Input: part model. Units: mm. Frame: model coordinates. Face numbers are marked on the shaded views. A direction names the side the tool comes from. Coordinates: 2 decimals unless noted, no trailing zeros. Write each loop counter-clockwise with the first axis right and the second up, starting at its lowest first coordinate (ties: lowest second). Pieces come first, ordered by that corner, then holes.
Autodesk Inventor part; units mm, degrees
ref_plane "YZ Plane" through (0, 0, 0) normal (1, 0, 0) x (0, 1, 0)
ref_plane "XZ Plane" through (0, 0, 0) normal (0, 1, 0) x (-1, 0, 0)
ref_plane "XY Plane" through (0, 0, 0) normal (0, 0, 1) x (1, 0, 0)
ref_plane "Work Plane1" through (0, 0, 0) normal (0, 0, 1) x (1, 0, 0)
sketch "Sketch1" plane through (0, 0, 0) normal (0, 0, 1) x (1, 0, 0)
  circle A0 centre (0, 25) radius 1.95 construction
  circle A1 centre (-25, 0) radius 1.95 construction
  circle A2 centre (-25, -25) radius 1.95 construction
  circle A3 centre (25, 25) radius 1.95 construction
  circle A4 centre (25, -25) radius 1.95 construction
  circle A5 centre (-25, 25) radius 1.95 construction
  circle A6 centre (25, 0) radius 1.95 construction
  circle A7 centre (0, -25) radius 1.95 construction
  line L0 (-28, 30) -> (-30, 28) construction
  line L1 (-30, 28) -> (-30, -28) construction
  line L2 (-30, -28) -> (-28, -30) construction
  line L3 (-28, -30) -> (28, -30) construction
  line L4 (28, -30) -> (30, -28) construction
  line L5 (30, -28) -> (30, 28) construction
  line L6 (30, 28) -> (28, 30) construction
  line L7 (28, 30) -> (-28, 30) construction
  circle A8 centre (35, -56) radius 1 construction
  circle A9 centre (5, -48.5) radius 1 construction
  circle A10 centre (5, -64.5) radius 1.0474 construction
  circle A11 centre (-5, -64.5) radius 1 construction
  circle A12 centre (-5, -56) radius 1 construction
  circle A13 centre (-5, -48.5) radius 1 construction
  circle A14 centre (5, -56) radius 1 construction
  circle A15 centre (35, -48) radius 1 construction
  circle A16 centre (35, -64) radius 1 construction
  line L8 (38, -40) -> (38, -72) construction
  line L9 (38, -40) -> (-10, -40) construction
  line L10 (-10, -72) -> (-10, -40) construction
  line L11 (38, -72) -> (-10, -72) construction
  line L12 (38, -71) -> (38, -41) construction
  line L13 (38, -71) -> (48, -71) construction
  line L14 (48, -41) -> (48, -71) construction
  line L15 (38, -41) -> (48, -41) construction
  line L16 (56, -75) -> (-52.5, -75)
  line L17 (-52.5, -75) -> (-52.5, -30)
  line L18 (-52.5, -30) -> (56, -30)
  line L19 (56, -30) -> (56, -75)
  line L20 (-40, -41.1445) -> (-40, -68) construction
  line L21 (-41, -39.0927) -> (-41, -47.7587) construction
  line L22 (-41, -39.0927) -> (-46.5, -39.0927) construction
  line L23 (-46.5, -47.7587) -> (-46.5, -39.0927) construction
  line L24 (-41, -47.7587) -> (-46.5, -47.7587) construction
  line L25 (-41, -60.5) -> (-41, -64) construction
  line L26 (-41, -60.5) -> (-46.5, -60.5) construction
  line L27 (-46.5, -64) -> (-46.5, -60.5) construction
  line L28 (-41, -64) -> (-46.5, -64) construction
  line L29 (64, 30) -> (-96, 30)
  line L30 (-96, 30) -> (-96, -80)
  line L31 (-96, -80) -> (64, -80)
  line L32 (64, -80) -> (64, 30)
  line L33 (20, -20) -> (-20, -20)
  line L34 (-20, -20) -> (-20, 20)
  line L35 (-20, 20) -> (20, 20)
  line L36 (20, 20) -> (20, -20)
  line L37 (20, -20) -> (-20, 20) construction
  line L38 (-20, -20) -> (20, 20) construction
  line L39 (-52.5, -30) -> (-30, -30)
  line L40 (-30, -30) -> (-30, -25)
  line L41 (-30, -25) -> (-52.5, -25)
  line L42 (-52.5, -25) -> (-52.5, -30)
  point P0 (0, 0)
  dimension "d1" = 3
  dimension "d2" = 8
  dimension "d4" = 6
  dimension "d5" = 160
  dimension "d6" = 110
  dimension "d7" = 8
  dimension "d19" = 40
  dimension "d20" = 40
  dimension "d28" = 5
  dimension "d29" = 0
extrude "Extrusion1" add sketch "Sketch1" along normal blind 10
sketch "Sketch2" plane through (0, 0, 10) normal (0, 0, 1) x (1, 0, 0)
  line L0 (-30, -30) -> (56, -30)
  line L1 (56, -30) -> (56, -75)
  line L2 (56, -75) -> (-52.5, -75)
  line L3 (64, 30) -> (-96, 30)
  line L4 (-96, 30) -> (-96, -80)
  line L5 (-96, -80) -> (64, -80)
  line L6 (64, -80) -> (64, 30)
  line L7 (20, -20) -> (20, 20)
  line L8 (-20, -20) -> (20, -20)
  line L9 (20, -20) -> (20, 20)
  line L10 (20, 20) -> (-20, 20)
  line L11 (-20, 20) -> (-20, -20)
  line L12 (-20, -20) -> (20, 20) construction
  line L13 (20, -20) -> (-20, 20) construction
  line L14 (-52.5, -25) -> (-30, -25)
  line L15 (-30, -25) -> (-30, -30)
  line L16 (-52.5, -75) -> (-52.5, -25)
  point P0 (0, 0)
extrude "Extrusion2" add sketch "Sketch2" along normal blind 4 contours L0 L1 L2 L16 L14 L15 | L6 L5 L4 L3
sketch "Sketch3" plane through (0, 0, 14) normal (0, 0, 1) x (1, 0, 0)
  circle A0 centre (0, 25) radius 1.95 construction
  circle A1 centre (-25, 0) radius 1.95 construction
  circle A2 centre (-25, -25) radius 1.95 construction
  circle A3 centre (25, 25) radius 1.95 construction
  circle A4 centre (25, -25) radius 1.95 construction
  circle A5 centre (-25, 25) radius 1.95 construction
  circle A6 centre (25, 0) radius 1.95 construction
  circle A7 centre (0, -25) radius 1.95 construction
  line L0 (-28, 30) -> (-30, 28) construction
  line L1 (-30, 28) -> (-30, -28) construction
  line L2 (-30, -28) -> (-28, -30) construction
  line L3 (-28, -30) -> (28, -30) construction
  line L4 (28, -30) -> (30, -28) construction
  line L5 (30, -28) -> (30, 28) construction
  line L6 (30, 28) -> (28, 30) construction
  line L7 (28, 30) -> (-28, 30) construction
  point P0 (0, 0)
hole "Hole1" at (25, 25, 14) at (0, 25, 14) at (-25, 25, 14) at (-25, 0, 14) at (-25, -25, 14) at (0, -25, 14) at (25, -25, 14) at (25, 0, 14) direction (0, 0, -1) diameter 3.3 end through all counterbore diameter 8 counterbore depth 5
sketch "Sketch4" plane through (0, 0, 0) normal (0, 0, -1) x (-1, 0, 0)
  line L0 (52.5, -75) -> (-56, -75) construction
  line L1 (-56, -75) -> (-56, -30) construction
  line L2 (-56, -30) -> (30, -30) construction
  line L3 (20, 20) -> (20, -20) construction
  line L4 (20, -20) -> (-20, -20) construction
  line L5 (-20, -20) -> (-20, 20) construction
  line L6 (-20, 20) -> (20, 20) construction
  line L7 (-64, 30) -> (96, 30) construction
  line L8 (-64, -80) -> (-64, 30) construction
  line L9 (96, -80) -> (-64, -80) construction
  line L10 (96, 30) -> (96, -80) construction
  line L11 (54.8114, -67.6244) -> (54.8114, -43.3756) construction
  line L12 (54.8114, -43.3756) -> (75.8114, -55.5) construction
  line L13 (75.8114, -55.5) -> (54.8114, -67.6244) construction
  line L14 (96, 30) -> (96, -80) construction
  line L15 (30, -30) -> (30, -25)
  line L16 (30, -25) -> (52.5, -25)
  line L17 (52.5, -25) -> (52.5, -75)
  line L18 (20, -49.5) -> (16.4, -49.5)
  line L19 (20, -61.5) -> (16.4, -61.5)
  circle A0 centre (5, -55.5) radius 1.8
  point P0 (0, 0)
  point P1 (61.8114, -55.5)
  dimension "d30" = 21
  dimension "d31" = 0
hole "Hole2" at (-54.8114, -43.3756, 0) at (-75.8114, -55.5, 0) at (-54.8114, -67.6244, 0) direction (0, 0, 1) diameter 2.8 depth 12 tip angle 118
sketch "Sketch5" plane through (0, 0, 14) normal (0, 0, 1) x (1, 0, 0)
  circle A0 centre (-75.8114, -55.5) radius 1.4
  circle A1 centre (-54.8114, -43.3756) radius 1.4
  circle A2 centre (-54.8114, -67.6244) radius 1.4
  circle A3 centre (25, -25) radius 1.65
  circle A4 centre (-25, -25) radius 1.65
  circle A5 centre (-25, 25) radius 1.65
  circle A6 centre (25, 25) radius 1.65
  circle A7 centre (0, 25) radius 1.65
  circle A8 centre (-25, 0) radius 1.65
  circle A9 centre (0, -25) radius 1.65
  circle A10 centre (25, 0) radius 1.65
  line L0 (64, 30) -> (-96, 30)
  line L1 (64, -80) -> (64, 30)
  line L2 (-96, -80) -> (64, -80)
  line L3 (-96, 30) -> (-96, -80)
  line L4 (-52.5, -25) -> (-52.5, -75)
  line L5 (-52.5, -75) -> (56, -75)
  line L6 (56, -75) -> (56, -30)
  line L7 (56, -30) -> (-30, -30)
  line L8 (-30, -30) -> (-30, -25)
  line L9 (-30, -25) -> (-52.5, -25)
  line L10 (-20, 20) -> (-20, -20)
  line L11 (-20, -20) -> (20, -20)
  line L12 (20, -20) -> (20, 20)
  line L13 (20, 20) -> (-20, 20)
  circle A11 centre (-75.8114, -55.5) radius 1.4
  circle A12 centre (-54.8114, -43.3756) radius 1.4
  circle A13 centre (-54.8114, -67.6244) radius 1.4
  point P0 (0, 0)
hole "Hole3" at (-54.8114, -43.3756, 14) at (-54.8114, -67.6244, 14) at (-75.8114, -55.5, 14) direction (0, 0, -1) diameter 2.9 depth 12 tip angle 118 counterbore diameter 7 counterbore depth 6
properties part number "cellSTORM_Base_v0"
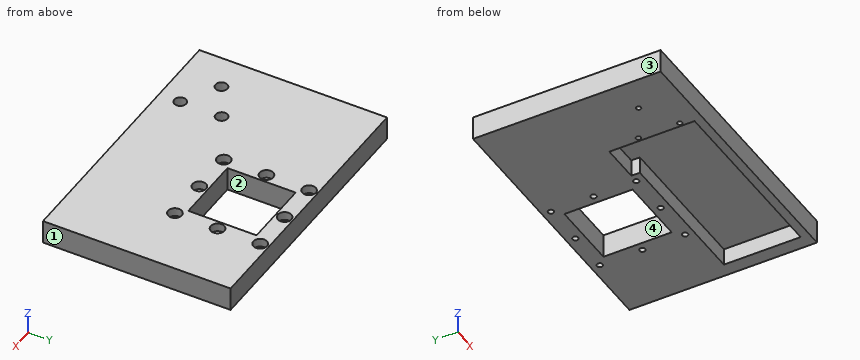
Item 1: Access query for the marked faces 1 and 2. Directions: +Z, -Z, +X, -X, +Y, -Y. A direction counts if a zero-diameter tool reaches every point of the face in a straight line with its end or side. Return the directions, or none.
Item 2: Pull-direction query (Y, two-part tool) for the marked faces 3 and 4; classes: released by +Y, released by -Y, zero draft, split by the parting line, or undercut.
Item 3: Material intervals for line 1 (Y direction, x = -11, z = 7); line 2 (X direction, y = 25, z = 2.5); line 3 (Y direction, x = 25, z = 12.85), sorted ascending.
Item 4: Section query C-C, the plane y = 25. Return loops of the section in (x, z).
Item 5: Section query B-B, the plane x = 25. State how many separate pieces and enclosed holes the cut face has, then the cut area to 3 significant figures.
Item 6: Pin query (flat end, axial travel): pin 1 Ø7 at (x, y) = (-25, 25) entering from +Z; pin 2 Ø4.5 at (x, y) = (-25, 25) entering from -Z; pin 3 Ø6.5 at (x, y) = (-54.81, -67.62) entering from +Z; pin 4 Ø1.7 at (x, y) = (-54.81, -43.38) entering from -Z. Return the tip coordinate at first contact, or that it passes through.
Item 7: Section query A-A, the plane y = 10. Return loops of the section in (x, z).
The answers:
1. face 1: +Z, -Z, +X, +Y, -Y
1. face 2: +Z, -Z
2. face 3: zero draft
2. face 4: undercut
3. line 1: y = -80 to -75, -30 to -20, 20 to 30
3. line 2: x = -96 to -26.65, -23.35 to -1.65, 1.65 to 23.35, 26.65 to 64
3. line 3: y = -80 to -29, -21 to -4, 4 to 21, 29 to 30
4. outline: (-96, 0) - (-26.65, 0) - (-26.65, 9) - (-29, 9) - (-29, 14) - (-96, 14) - close; (-23.35, 0) - (-1.65, 0) - (-1.65, 9) - (-4, 9) - (-4, 14) - (-21, 14) - (-21, 9) - (-23.35, 9) - close; (1.65, 0) - (23.35, 0) - (23.35, 9) - (21, 9) - (21, 14) - (4, 14) - (4, 9) - (1.65, 9) - close; (26.65, 0) - (64, 0) - (64, 14) - (29, 14) - (29, 9) - (26.65, 9) - close
5. separate pieces: 4
5. enclosed holes: 0
5. area: 881 mm2
6. pin 1: stops at z = 9
6. pin 2: stops at z = 0
6. pin 3: stops at z = 8
6. pin 4: passes through
7. outline: (-96, 0) - (-20, 0) - (-20, 14) - (-96, 14) - close; (20, 0) - (64, 0) - (64, 14) - (20, 14) - close
